Could you check a few things on this drawing? It's one solid part, dimensions in mm from its lowest x, y, z. A direction names the side the tool comes from. Round coordinates to 2 decimals unless told otherwise and drop trailing zeros. Order: outer loops, then holes, each group sorted by start corner. A loop starts at its lowest first (then second) coordinate and runs counter-clockwise, first axis right, second up. Notation, with made-up numbers: (30.25, 79.5) - (47.25, 79.5) arc R8 cw to (47.25, 89.5) - close; hole circle Ø3 at (4.5, 37.25). An arc over 180 degrees is marked (long way). Use one line per item in the form item = value.
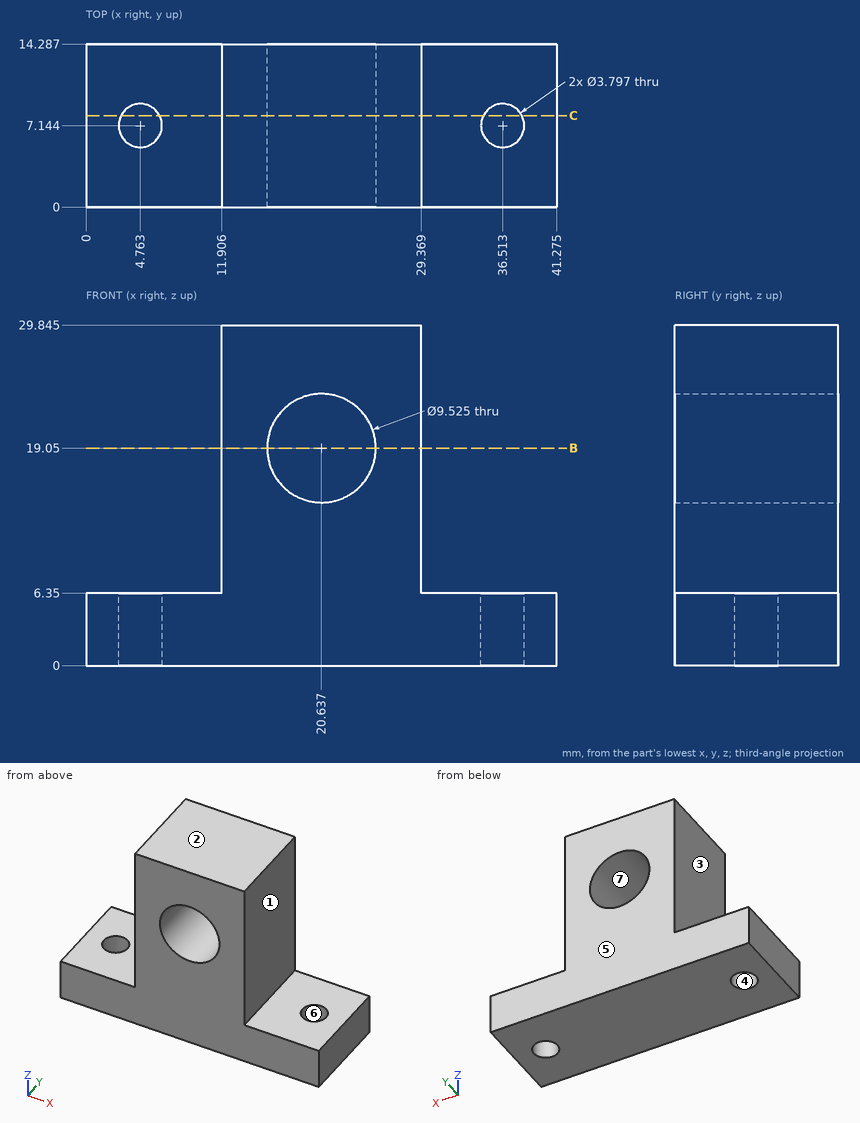
Item 1: I need wall thicknesses on L1, parallel to Z at x = 20.5, y = 12.5 (1 decimal); L2, parallel to X at y = 8.25, z = 6 (1 decimal); L3, parallel to X at y = 8.5, z = 3 (1 decimal). Which ranges of each line are inside material? Lowest first, please.
Found:
L1 = 0 to 14.3, 23.8 to 29.8
L2 = 0 to 3.2, 6.3 to 35, 38.1 to 41.3
L3 = 0 to 3.4, 6.1 to 35.2, 37.8 to 41.3
Item 2: If we mould it in two halves opening along Y, with no side actions, what happens to the marked faces 4, 5, 6 and 7? For each: released by +Y, released by -Y, zero draft, split by the parting line, or undercut.
Found:
face_4 = undercut
face_5 = released by +Y
face_6 = undercut
face_7 = zero draft
Item 3: Will these pins go through, and if not, where does the flat tip stop? P1, Ø1, axis at y = 12.5, z = 12.5, coming from the +X side; P2, Ø12, axis at x = 5.5, z = 12.5, coming from the -Y side; P3, Ø3.5, axis at x = 4.5, y = 9.5, coming from the +Z side.
Found:
P1 = 29.37
P2 = through
P3 = 6.35
Item 4: Imagine slicing it at B-B on z = 19.05. Please give me the cut outline in (x, y) (1 decimal), plus the area to 3 significant figures.
Found:
outline = (11.9, 0) - (15.9, 0) - (15.9, 14.3) - (11.9, 14.3) - close; (25.4, 0) - (29.4, 0) - (29.4, 14.3) - (25.4, 14.3) - close
area = 113 mm2
Item 5: Imagine slicing it at C-C on y = 8. State how many separate pieces and enclosed holes the cut face has, plus the area to 3 significant figures.
Found:
separate_pieces = 3
enclosed_holes = 1
area = 558 mm2
Item 6: For the marked faces 1, 2 and 3, which set-ups out of +Z, -Z, +X, -X, +Y, -Y let a thin tool reach every point of the face, with its end or its side?
Found:
face_1 = +Z, +X, +Y, -Y
face_2 = +Z, +X, -X, +Y, -Y
face_3 = +Z, -X, +Y, -Y
